Here's how the part is built. I have some questions about the finished solid (model axes, mm). Face numbers are marked on the shaded views. A direction names the side the tool comes from. Give positions to 0.01 mm unless a question says otherwise; leave off trailing zeros.
Q1. I need wall thicknesses on line 1 (Y direction, x = -7, z = 9.5); line 2 (X direction, y = -24, z = 15.25); line 3 (X direction, y = -2.5, z = 3.5). Which ranges of each line are inside material? Lowest first, please.
Q2. If we section it at C-C (z = 10.75): Give the number of separate pieces and of enclosed holes in the cut face, plus the area to 3 significant figures.
Q3. For the marked faces 1 and 2, which set-ups out of +Z, -Z, +X, -X, +Y, -Y let a thin tool reach every point of the face, with its end or its side?
Q4. We'd pull the mould along X, two halves only. Please class the marked faces 3, 4, 5 and 6: +X half, -X half, draft (parallel to the pull), parting line (faces both ways), or undercut.
Q5. Will this pin go through, and if not, where does the flat tip stop? P1, Ø19, axis at x = 52.5, y = -20.5, coming from the +Z side.
from build123d import *

# Parameters (mm, degrees)
F0_W         = 150
F0_H         = 88.883145673
F1_DEPTH     = 20
F2_W         = 142
F2_H         = 80.883145673
F3_DEPTH     = 19
F5_DEPTH     = 16
F6_R         = 1.99999
F7_T1_DEPTH  = 63.6293265809
F7_T3_DEPTH  = 34.4415928365
F7_T5_DEPTH  = 34.4415928365
F7_T8_ANGLE  = 90
F7_T10_ANGLE = 90
F7_T14_ANGLE = 163.703254406
F7_T19_ANGLE = 163.703254406
F7_T24_ANGLE = 163.703254406
F7_T29_ANGLE = 163.703254406


# Not quite as in the source:
# - a fillet or chamfer that OpenCascade refuses, or shapes differently, is made with other operations: its cross-section is extruded or revolved along the edge and cut away or added
# - a fillet or chamfer is up to 0.001 mm smaller than in the source, because OpenCascade refuses the exact size
# - a feature names something its author has since deleted; it is built from what else it names


with BuildPart() as f1:
    # F0 (on Top) → F1 (new body)
    with BuildSketch(Plane.XY):
        Rectangle(F0_W, F0_H)
    extrude(amount=F1_DEPTH)

    # F2 (on face) → F3 (cut)
    with BuildSketch(Plane.XY.offset(20)):
        Rectangle(F2_W, F2_H)
    extrude(amount=-F3_DEPTH, mode=Mode.SUBTRACT)

    # F4 (on face) → F5 (join)
    with BuildSketch(Plane.XY.offset(1)):
        Polygon((3.3706934191, -2), (71, -2), (71, 2), (3.3706934191, 2), (3.3706934191, 40.4415728365), (-1.4311365085, 40.4415728365), (-1.4311365085, 2), (-71, 2), (-71, -2), (-1.4311365085, -2), (-1.4311365085, -40.4415728365), (3.3706934191, -40.4415728365), align=None)
    extrude(amount=F5_DEPTH)

    # F6 (radius 2 in the source; OpenCascade refuses exactly that, so slightly less here)
    f6_edges = [f1.edges().sort_by_distance(p)[0] for p in [
        (-75, 0, 20),
        (0, 44.441573, 20),
        (0, -44.441573, 20),
        (75, 0, 20),
        (-75, -44.441573, 10),
        (-75, 44.441573, 10),
        (75, -44.441573, 10),
        (75, 44.441573, 10),
        (0, 44.441573, 0),
        (-71, -40.441573, 10.5),
        (-71, 40.441573, 10.5),
        (71, -40.441573, 10.5),
        (71, 40.441573, 10.5),
        (71, 2, 9),
        (71, -2, 9),
        (71, 0, 20),
        (0, 40.441573, 20),
        (0, -40.441573, 20),
        (-71, 0, 20),
        (-1.431137, 2, 9),
        (3.370693, 2, 9),
        (-1.431137, -2, 9),
        (-1.431137, 40.441573, 9),
        (3.370693, 40.441573, 9),
        (-71, -2, 9),
        (-71, 2, 9),
        (3.370693, -40.441573, 9),
        (-1.431137, -40.441573, 9),
        (3.370693, -2, 9),
    ]]
    fillet(f6_edges, radius=F6_R)

    # F7: chamfer of 1 on 6 edges, made by hand

    # F7_s2 → F7_t1 (cut)
    with BuildSketch(Plane.YZ.offset(5.3706834191)):
        Polygon((1, 17), (2, 16), (2, 17), align=None)
        Polygon((-1, 17), (-2, 16), (-2, 17), align=None)
    extrude(amount=F7_T1_DEPTH, mode=Mode.SUBTRACT)

    # F7_s4 → F7_t3 (cut)
    with BuildSketch(Plane.XZ.offset(3.99999)):
        Polygon((2.3706934191, 17), (3.3706934191, 16), (3.3706934191, 17), align=None)
    extrude(amount=F7_T3_DEPTH, mode=Mode.SUBTRACT)

    # F7_s6 → F7_t5 (cut)
    with BuildSketch(Plane.XZ.offset(-38.4415828365)):
        Polygon((2.3706934191, 17), (3.3706934191, 16), (3.3706934191, 17), align=None)
    extrude(amount=F7_T5_DEPTH, mode=Mode.SUBTRACT)

    # F7_s7 → F7_t8 (revolve, cut)
    with BuildSketch(Plane.XZ.offset(3.99999)):
        Polygon((2.3706934191, 17), (3.3706934191, 16), (3.3706934191, 17), align=None)
    revolve(axis=Axis((5.3706834191, -3.99999, 17), (0, 0, -1)), revolution_arc=F7_T8_ANGLE, mode=Mode.SUBTRACT)

    # F7_s9 → F7_t10 (revolve, cut)
    with BuildSketch(Plane.YZ.offset(5.3706834191)):
        Polygon((1, 17), (2, 16), (2, 17), align=None)
    revolve(axis=Axis((5.3706834191, 3.99999, 17), (0, 0, -1)), revolution_arc=F7_T10_ANGLE, mode=Mode.SUBTRACT)


with BuildPart() as f7_tool12:
    # F7_s13 → F7_t14 (revolve)
    with BuildSketch(Plane(origin=(-9.930856522, 33.9680428578, 0), x_dir=(0, 0, 1), z_dir=(0.2806121914, -0.9598212323, 0))):
        Polygon((17, -18.9420627796), (16, -17.9420627796), (17, -17.9420627796), align=None)
    revolve(axis=Axis((5.3706834191, 38.4415828365, 17), (0, 0, 1)), revolution_arc=F7_T14_ANGLE)

    split(bisect_by=Plane.XZ.offset(-40.4415728365), keep=Keep.TOP)


with BuildPart() as f1_1:
    add(f1.part)

    # F7_t11: cut F7_tool12
    add(f7_tool12.part, mode=Mode.SUBTRACT)


with BuildPart() as f7_tool17:
    # F7_s18 → F7_t19 (revolve)
    with BuildSketch(Plane(origin=(-9.930856522, -33.9680428578, 0), x_dir=(0, 0, 1), z_dir=(0.2806121914, 0.9598212323, 0))):
        Polygon((17, 18.9420627796), (16, 17.9420627796), (17, 17.9420627796), align=None)
    revolve(axis=Axis((5.3706834191, -38.4415828365, 17), (0, 0, -1)), revolution_arc=F7_T19_ANGLE)

    split(bisect_by=Plane.XZ.offset(40.4415728365), keep=Keep.BOTTOM)


with BuildPart() as f1_2:
    add(f1_1.part)

    # F7_t16: cut F7_tool17
    add(f7_tool17.part, mode=Mode.SUBTRACT)


with BuildPart() as f7_tool22:
    # F7_s23 → F7_t24 (revolve)
    with BuildSketch(Plane(origin=(62.4893808118, 18.2693208905, 0), x_dir=(0, 0, 1), z_dir=(-0.9598212323, -0.2806121914, 0))):
        Polygon((17, -26.201509346), (16, -25.201509346), (17, -25.201509346), align=None)
    revolve(axis=Axis((69.00001, -3.99999, 17), (0, 0, 1)), revolution_arc=F7_T24_ANGLE)

    split(bisect_by=Plane.YZ.offset(71), keep=Keep.BOTTOM)


with BuildPart() as f1_3:
    add(f1_2.part)

    # F7_t21: cut F7_tool22
    add(f7_tool22.part, mode=Mode.SUBTRACT)


with BuildPart() as f7_tool27:
    # F7_s28 → F7_t29 (revolve)
    with BuildSketch(Plane(origin=(62.4893808118, -18.2693208905, 0), x_dir=(0, 0, 1), z_dir=(-0.9598212323, 0.2806121914, 0))):
        Polygon((16, 25.201509346), (17, 26.201509346), (17, 25.201509346), align=None)
    revolve(axis=Axis((69.00001, 3.99999, 17), (0, 0, -1)), revolution_arc=F7_T29_ANGLE)

    split(bisect_by=Plane.YZ.offset(71), keep=Keep.BOTTOM)


with BuildPart() as f1_4:
    add(f1_3.part)

    # F7_t26: cut F7_tool27
    add(f7_tool27.part, mode=Mode.SUBTRACT)


solid = f1_4.part
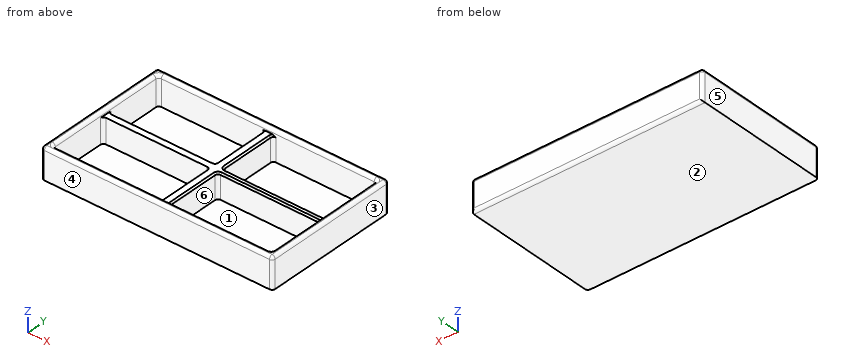
Check sheet entries:
1. line 1: y = -44.44 to -40.44, -2 to 2, 40.44 to 44.44
1. line 2: x = -75 to -71, -1.43 to 3.37, 71 to 75
1. line 3: x = -75 to -70.32, -2.11 to 4.05, 70.32 to 75
2. separate pieces: 1
2. enclosed holes: 4
2. area: 2,790 mm2
3. face 1: +Z
3. face 2: -Z, +X, -X, +Y, -Y
4. face 3: +X half
4. face 4: draft
4. face 5: -X half
4. face 6: undercut
5. P1: stops at z = 1
